```python
from build123d import *

# Parameters (mm, degrees)
BOSS_EXTRUDE1_DEPTH = 1.7
SKETCH2_R           = 2.35
BOSS_EXTRUDE2_DEPTH = 4.7
FILLET1_R           = 3
SKETCH3_R           = 2.4
CUT_EXTRUDE1_DEPTH  = 1


with BuildPart() as part:
    # Sketch1 → Boss-Extrude1 (new body)
    with BuildSketch(Plane(origin=(0, 0, 0), x_dir=(1, 0, 0), z_dir=(0, 1, 0))):
        Polygon((0, 0), (0, 80), (37.3, 80), (37.3, 75), (17, 75), (17, 0), align=None)
    extrude(amount=BOSS_EXTRUDE1_DEPTH)

    # Sketch2 → Boss-Extrude2 (add)
    with BuildSketch(Plane(origin=(0, 0, 0), x_dir=(-1, 0, 0), z_dir=(0, -1, 0))):
        with Locations(Location((-13.25, 10, 0), (0, 0, 90))):
            Circle(SKETCH2_R)
        with Locations(Location((-8, 72, 0), (0, 0, 90))):
            Circle(SKETCH2_R)
    extrude(amount=BOSS_EXTRUDE2_DEPTH)

    # Fillet1
    fillet1_edges = [part.edges().sort_by_distance(p)[0] for p in [
        (0, 0.85, -80),
    ]]
    fillet(fillet1_edges, radius=FILLET1_R)

    # Sketch3 → Cut-Extrude1 (cut)
    with BuildSketch(Plane(origin=(0, 0, 0), x_dir=(-1, 0, 0), z_dir=(0, -1, 0))):
        with Locations(Location((-13.25, 61.25, 0), (0, 0, 90))):
            Circle(SKETCH3_R)
    extrude(amount=-CUT_EXTRUDE1_DEPTH, mode=Mode.SUBTRACT)

    # Mirror3: part across plane


with BuildPart() as part_1:
    add(part.part)
    add(part.part.mirror(Plane(origin=(37.3, 1.7, -80), x_dir=(0, 0, 1), z_dir=(-1, 0, 0))))


solid = part_1.part
```
Here's how the part is built. I have some questions about the finished solid (model axes, mm). A direction names the side the tool comes from. Give positions to 0.01 mm unless a question says otherwise; leave off trailing zeros. Loops run counter-clockwise (first coordinate to the right, second up) from the corner with the lowest first, then second, coordinate; pieces in that order, holes last. Notation, with made-up numbers: M 18.5,10.5 L 54.5,10.5 A3 ccw 54.5,15.5 Z; hole C 18.5,58 d8. An arc over 180 degrees is marked long. Put each result on its own line as item: value. Start each with the question number.
(1) For faces 1 (the flat face through (66, 1, 0)), 2 (the cylindrical face through (64.27, -2.32, -71.69)), 3 (the flat face through (17, 1, -38)), which set-ups out of +Z, -Z, +X, -X, +Y, -Y let a thin tool reach every point of the face, with its end or its side?
(2) I want a section at D-D on z = -18.5. Please give me the cut outline in (x, y).
(3) I want a section at C-C on y = -3.75. Please give me the cut outline in (x, z), then the cut area to 3 significant figures.
(4) I need wall thicknesses on line 1 along X through (y, z) = (0.45, -61.25); line 2 along X through (y, z) = (1, -23); line 3 along Z through (x, y) = (61.35, 0.6). Which ranges of each line are inside material? Lowest first, please. Write a range as [from, to].
(5) Will these pins go through, and if not, where does the flat tip stop? pin 1 Ø2.5 at (x, z) = (14.5, -61.5) entering from -Y; pin 2 Ø1.9 at (x, y) = (40, 0.5) entering from +Z; pin 3 Ø2.5 at (x, z) = (62, -62) entering from -Y.
(6) If we mould it in two halves opening along X, with no side actions, what happens to faces 4 (the cylindrical face through (73.74, 0.86, -79.1)), 5 (the flat face through (57.6, 1, -38)), 6 (the flat face through (8, -4.7, -72))? For each: +X half, -X half, draft (parallel to the pull), parting line (faces both ways), or undercut.
(7) I want a section at B-B on x = 66.6. Please give me the cut outline in (y, z).
(8) I want a section at A-A on z = -72. Please give me the cut outline in (x, y), then the cut area to 3 significant figures.
Answer block:
1. face 1: +Z, +X, -X, +Y, -Y
1. face 2: -Y
1. face 3: +Z, +Y, -Y
2. outline: M 0,0 L 17,0 L 17,1.7 L 0,1.7 Z; M 57.6,0 L 74.6,0 L 74.6,1.7 L 57.6,1.7 Z
3. outline: C 8,-72 d4.7; C 13.25,-10 d4.7; C 61.35,-10 d4.7; C 66.6,-72 d4.7
3. area: 69.4 mm^2
4. line 1: [0, 10.85], [15.65, 17], [57.6, 58.95], [63.75, 74.6]
4. line 2: [0, 17], [57.6, 74.6]
4. line 3: [-80, -63.65], [-58.85, 0]
5. pin 1: y = 0
5. pin 2: z = -75
5. pin 3: y = 1
6. face 4: +X half
6. face 5: undercut
6. face 6: draft
7. outline: M -4.7,-74.35 L 0,-74.35 L 0,-80 L 1.7,-80 L 1.7,0 L 0,0 L 0,-69.65 L -4.7,-69.65 Z
8. outline: M 0,0 L 5.65,0 L 5.65,-4.7 L 10.35,-4.7 L 10.35,0 L 17,0 L 17,1.7 L 0,1.7 Z; M 57.6,0 L 64.25,0 L 64.25,-4.7 L 68.95,-4.7 L 68.95,0 L 74.6,0 L 74.6,1.7 L 57.6,1.7 Z
8. area: 102 mm^2
